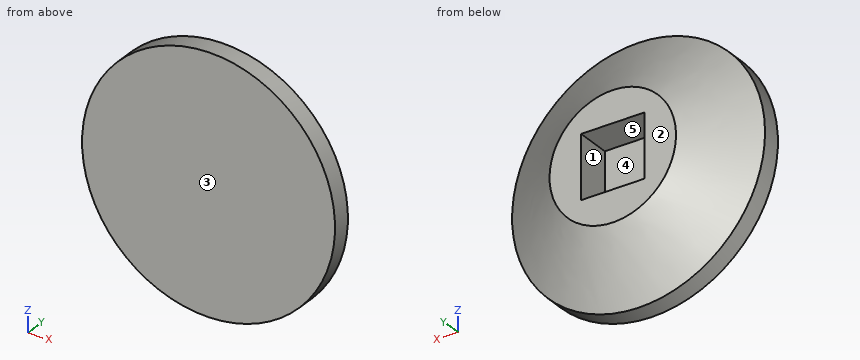
```python
from build123d import *

# Parameters (mm, degrees)
SKETCH1_R           = 20
BOSS_EXTRUDE1_DEPTH = 1.5
SKETCH5_W           = 10
SKETCH5_H           = 10
CUT_EXTRUDE1_DEPTH  = 5.5


with BuildPart() as part:
    # Sketch1 → Boss-Extrude1 (new, symmetric)
    with BuildSketch(Plane(origin=(0, 0, 0), x_dir=(1, 0, 0), z_dir=(0, 1, 0))):
        with Locations(Location((0, 0, 0), (0, 0, 270))):
            Circle(SKETCH1_R)
    extrude(amount=BOSS_EXTRUDE1_DEPTH, both=True)

    # Loft1: read off the stored shape, not the designer's step
    # Loft1: loft between two sections, ruled curve by curve
    loft1_from = [
        Edge.make_bspline([(-6.427341281, 7.5, -7.660893163), (8.894445045, 7.5, -20.515575726), (21.749127607, 7.5, -5.1937894), (6.427341281, 7.5, 7.660893163), (-8.894445045, 7.5, 20.515575726), (-21.749127607, 7.5, 5.1937894), (-6.427341281, 7.5, -7.660893163)], [0, 0, 0, 0, 0.5, 0.5, 0.5, 1, 1, 1, 1], 3, [1, 0.333333333, 0.333333333, 1, 0.333333333, 0.333333333, 1]),
    ]
    loft1_to = [
        Edge.make_bspline([(-15.74903345, 1.5, -12.327527951), (8.906022452, 1.5, -43.825594852), (40.404089352, 1.5, -19.17053895), (15.74903345, 1.5, 12.327527951), (-8.906022452, 1.5, 43.825594852), (-40.404089352, 1.5, 19.17053895), (-15.74903345, 1.5, -12.327527951)], [0, 0, 0, 0, 0.5, 0.5, 0.5, 1, 1, 1, 1], 3, [1, 0.333333333, 0.333333333, 1, 0.333333333, 0.333333333, 1]),
    ]
    loft1 = Solid(Shell([*[Face.make_surface_from_curves(loft1_from[k], loft1_to[k]) for k in range(1)], Face(Wire(loft1_from)), Face(Wire(loft1_to))]))
    add(loft1)

    # Sketch5 → Cut-Extrude1 (cut)
    with BuildSketch(Plane(origin=(0, 7.5, 0), x_dir=(1, 0, 0), z_dir=(0, 1, 0))):
        Rectangle(SKETCH5_W, SKETCH5_H)
    extrude(amount=-CUT_EXTRUDE1_DEPTH, mode=Mode.SUBTRACT)


solid = part.part
```
Work out the finished part from the listing and answer in its coordinate system (mm). Face numbers are marked on the shaded views. A direction names the side the tool comes from. Give positions to 0.01 mm unless a question says otherwise; leave off trailing zeros. Write each loop counter-clockwise with the first axis right and the second up, starting at its lowest first coordinate (ties: lowest second). Pieces come first, ordered by that corner, then holes.
(1) Flat-ended cylindrical pins translate along their axes: pin 1 Ø2 at (x, z) = (1, 3) entering from +Y; pin 2 Ø1 at (x, y) = (-13.5, 1) entering from -Z; pin 3 Ø4.5 at (x, y) = (-1.5, 5) entering from +Z. Find the tip coordinate at first contact, or state that the pin passes through.
Final values:
pin 1: stops at y = 2
pin 2: stops at z = -15.2
pin 3: stops at z = 17.82
(2) Which of the six approach directions +Z, -Z, +X, -X, +Y, -Y give full straight-line access (tool end or side, diameter ignored) to the marked faces 1 and 2?
Final values:
face 1: +Y
face 2: +Z, -Z, +X, -X, +Y
(3) Straight lines are drawn through the part: line 1 (X direction, y = 2.5, z = 1.5); line 2 (Z direction, x = 1, y = 5.75); line 3 (Z direction, x = -0.5, y = 5). For each, find the intervals that lie inside material, in ascending order.
Final values:
line 1: x = -18.24 to -5, 5 to 18.24
line 2: z = -12.81 to -5, 5 to 12.81
line 3: z = -14.08 to -5, 5 to 14.08
(4) The part is cut by section A-A on y = -1. Write down the section's boundary in (x, z), plus the area to 3 significant figures.
Final values:
outline: circle Ø40 at (0, 0)
area: 1,260 mm2
(5) The mould has two halves that part along Z. Classify the marked faces 3, 4 and 5: pulls with the +Z half, pulls with the -Z half, needs draft (parallel to the pull), parting line crosses it, or undercut.
Final values:
face 3: needs draft
face 4: undercut
face 5: undercut
